from build123d import *

# Parameters (mm, degrees)
BOSS_EXTRUDE1_DEPTH = 2.25
FILLET1_R           = 5
FILLET2_R           = 3
SKETCH2_R           = 1.75
CUT_EXTRUDE1_DEPTH  = 47.840102946
BOSS_EXTRUDE2_REACH = 40.51
SKETCH4_W           = 6.5
SKETCH4_H           = 2.1
BOSS_EXTRUDE3_REACH = 40.51
SKETCH4_2_W         = 6.5
SKETCH4_2_H         = 2.1


with BuildPart() as part:
    # Sketch1 → Boss-Extrude1 (new body)
    with BuildSketch(Plane(origin=(0, 0, 0), x_dir=(1, 0, 0), z_dir=(0, 1, 0))):
        Polygon((0, 0), (9.957880591, 14.994686196), (15.4441772, 42.451935686), (20.033915457, 42.451935686), (17.6175711, 12.686192897), (7.659690509, -2.308493299), align=None)
    extrude(amount=BOSS_EXTRUDE1_DEPTH)

    # Fillet1
    # the kernel refuses this fillet: 5 mm, written as the material it takes off along each edge
    with BuildSketch(Plane(origin=(7.659690509, -9.280606122, 2.308493299), x_dir=(0.5532155884096079, 0, -0.8330381220212022), z_dir=(0, 1, 0))) as fillet1_piece_1:
        with BuildLine():
            CenterArc((FILLET1_R * 0.742448489754, FILLET1_R), FILLET1_R, 196.816032259, 73.183967741)
            Line((-FILLET1_R * 0.214790094662, FILLET1_R * 0.710700341335), (0, 0))
            Line((0, 0), (FILLET1_R * 0.742448489754, 0))
        make_face()
    extrude(amount=20.811212244, mode=Mode.SUBTRACT)
    with BuildSketch(Plane(origin=(0, -16.83618483, 0), x_dir=(0.5532155884096086, 0, -0.8330381220212018), z_dir=(0, 1, 0))) as fillet1_piece_2:
        with BuildLine():
            CenterArc((FILLET1_R * 1.34689478637, -FILLET1_R), FILLET1_R, 90, 106.816032259)
            Line((FILLET1_R * 0.389656201955, -FILLET1_R * 1.28929965867), (0, 0))
            Line((0, 0), (FILLET1_R * 1.34689478637, 0))
        make_face()
    extrude(amount=35.922369659, mode=Mode.SUBTRACT)

    # Fillet2
    # the kernel refuses this fillet: 3 mm, written as the material it takes off along each edge
    with BuildSketch(Plane(origin=(15.4441772, -6.149660967, -42.451935686), x_dir=(-0.19593916459228597, 0, 0.9806160531925209), z_dir=(0, 1, 0))) as fillet2_piece_1:
        with BuildLine():
            CenterArc((FILLET2_R * 0.819954795549, FILLET2_R), FILLET2_R, 191.29959219, 78.70040781)
            Line((-FILLET2_R * 0.160661257643, FILLET2_R * 0.804060835408), (0, 0))
            Line((0, 0), (FILLET2_R * 0.819954795549, 0))
        make_face()
    extrude(amount=14.549321933, mode=Mode.SUBTRACT)
    with BuildSketch(Plane(origin=(20.033915457, -8.133512114, -42.451935686), x_dir=(-0.08091253350556188, 0, 0.9967212057148735), z_dir=(0, 1, 0))) as fillet2_piece_2:
        with BuildLine():
            CenterArc((FILLET2_R * 1.08446828191, -FILLET2_R), FILLET2_R, 90, 94.641020106)
            Line((FILLET2_R * 0.0877470761958, -FILLET2_R * 1.08091253351), (0, 0))
            Line((0, 0), (FILLET2_R * 1.08446828191, 0))
        make_face()
    extrude(amount=18.517024229, mode=Mode.SUBTRACT)

    # Sketch2 → Cut-Extrude1 (cut, through all)
    with BuildSketch(Plane(origin=(0, 2.25, 0), x_dir=(1, 0, 0), z_dir=(0, 1, 0))):
        with Locations(Location((8.353327454, 5.514543703, 0), (0, 0, 270))):
            Circle(SKETCH2_R)
        with Locations(Location((14.060025472, 18.298658758, 0), (0, 0, 270))):
            Circle(SKETCH2_R)
    extrude(amount=-CUT_EXTRUDE1_DEPTH, mode=Mode.SUBTRACT)

    # Boss-Extrude2: up to this plane
    boss_extrude2_end = Plane(origin=(17.6175711, 2.25, -12.686192897), z_dir=(-0.9967212057148735, 0, -0.0809125335055623))
    # Sketch4 → Boss-Extrude2 (add, up to the surface)
    with BuildSketch(Plane(origin=(20.2, -1.484709168, -8.201879583), x_dir=(0, 0, -1), z_dir=(1, 0, 0)), mode=Mode.PRIVATE) as boss_extrude2_sk1:
        with Locations((28.408493587, 2.541926215)):
            Rectangle(SKETCH4_W, SKETCH4_H)
    boss_extrude2_tool1 = split(extrude(boss_extrude2_sk1.sketch, amount=-BOSS_EXTRUDE2_REACH, mode=Mode.PRIVATE), bisect_by=boss_extrude2_end, keep=Keep.BOTH, mode=Mode.PRIVATE)
    add(boss_extrude2_tool1.solids().sort_by_distance((20.2, 1.057217, -36.610373))[0])

    # Boss-Extrude3: up to this face of the body (flat: up to its plane)
    boss_extrude3_end = Plane(part.part.faces().sort_by_distance((18.476650911, 1.142566407, -23.268769271))[0])
    # Sketch4<2> → Boss-Extrude3 (add, up to the picked face)
    with BuildSketch(Plane(origin=(20.2, -1.484709168, -8.201879583), x_dir=(0, 0, -1), z_dir=(1, 0, 0)), mode=Mode.PRIVATE) as boss_extrude3_sk1:
        with Locations((28.408493587, 2.541926215)):
            Rectangle(SKETCH4_2_W, SKETCH4_2_H)
    boss_extrude3_tool1 = split(extrude(boss_extrude3_sk1.sketch, amount=-BOSS_EXTRUDE3_REACH, mode=Mode.PRIVATE), bisect_by=boss_extrude3_end, keep=Keep.BOTH, mode=Mode.PRIVATE)
    add(boss_extrude3_tool1.solids().sort_by(Axis((20.2, 1.057217, -36.610373), (-1, 0, 0)))[0])


solid = part.part
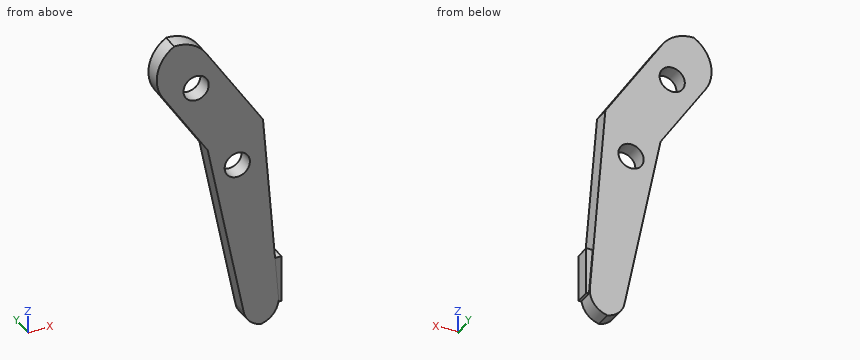
Build history of the part. All positions in model axes, mm. Coordinates: 2 decimals unless noted, no trailing zeros. Order: outer loops, then holes, each group sorted by start corner. A loop starts at its lowest first (then second) coordinate and runs counter-clockwise, first axis right, second up. Notation, with made-up numbers: M 3,38 L 59,38 A38 cw 59,76 Z; hole C 41,-40 d1. An arc over 180 degrees is marked long. One line per question, with ' | ' between items. Start each with the question number.
Q1. Saw through at B-B (y = 0.8). List the corners of the cut face in (x, z), then the cut area to 3 significant figures.
Q2. Saw through at A-A (x = 7.25). List the corners of the cut face in (y, z), then the cut area to 3 significant figures.
Q3. Probe L1, parallel to X at y = 0.15, z = -17; L2, parallel to X at y = 0.9, z = -6; L3, parallel to Z at x = 17, y = 1.75. List the from-to ranges inside material, lowest first. Write a range as from..to.
Q4. Flat gauge pins, fed straight in: pin 1 Ø0.7 at (x, z) = (19.5, -35) entering from +Y; pin 2 Ø0.7 at (x, y) = (20, 1) entering from +Z. Where does each tip first touch, or does it go through?
Q5. Saw through at D-D (x = 9.25). List the corners of the cut face in (y, z).
Check values:
1) outline: M 3.73,-5.61 L 9.96,-14.99 L 14.96,-40.04 A3 ccw 17.34,-42.4 A3 ccw 19.77,-39.21 L 19.82,-39.86 L 20.2,-39.86 L 20.2,-33.36 L 19.3,-33.36 L 17.62,-12.69 L 9.71,-0.78 A5 ccw 5.32,1.44 A5 ccw Z; hole C 8.35,-5.51 d3.5; hole C 14.06,-18.3 d3.5 | area: 286 mm2
2) outline: M 0,-10.92 L 2.25,-10.92 L 2.25,-6.87 L 0,-6.87 Z; M 0,-4.16 L 2.25,-4.16 L 2.25,1.15 L 0,1.15 Z | area: 21.0 mm2
3) L1: x = 10.36..12.89, 15.23..17.97 | L2: x = 3.98..6.67, 10.03..13.18 | L3: z = -42.31..-11.76
4) pin 1: stops at y = 2.25 | pin 2: stops at z = -33.36
5) outline: M 0,-13.93 L 2.25,-13.93 L 2.25,-7.02 L 0,-7.02 Z; M 0,-4.01 L 2.25,-4.01 L 2.25,-0.19 L 0,-0.19 Z
